Read the model definition and answer for the solid it produces. Units are mm, in the model's axes. A direction names the side the tool comes from. Round coordinates to 2 decimals unless told otherwise and drop trailing zeros. Order: outer loops, then holes, each group sorted by start corner. A loop starts at its lowest first (then second) coordinate and runs counter-clockwise, first axis right, second up. Notation, with made-up numbers: (-13.5, -34.75) - (8.5, -34.75) arc R36 ccw to (8.5, 2.25) - close; hole circle Ø5 at (63, 32). An arc over 180 degrees is marked (long way). One line per question, with ' | ' between items. Start each with the question number.
1) For faces 4 (the flat face through (368, 71, 95)), 5 (the cylindrical face through (377.75, 40.77, 85.56)), determine the directions among +Z, -Z, +X, -X, +Y, -Y from which every point of the face is accessible in a straight line to the end or side of a thin tool.
2) Straight lines are drawn through the part: line 1 (Z direction, x = 378.25, y = 114.8); line 2 (Y direction, x = 377.5, z = 13.2); line 3 (Z direction, x = 372.75, y = 40.7). For each, find the intervals that lie inside material, in ascending order. Write a range as from..to.
3) The part is cut by section A-A, the plane y = 114.8. Give the vertices of the cut face in (x, z), plus the area to 3 significant figures.
4) The mould has two halves that part along Y. Classify faces 1 (the flat face through (368, 22.5, 52)), 2 (the cylindrical face through (377.746, 116.426, 12.987)), 3 (the flat face through (388, 71, 53)): pulls with the +Y half, pulls with the -Y half, needs draft (parallel to the pull), parting line crosses it, or undercut.
5) The part is cut by section B-B, the plane z = 13.2. Give the vertices of the cut face in (x, y).
6) A flat-ended cylindrical pin translates along its axis: pin 1 (3 mm diameter, centred on y = 114.8, z = 13.2, fed in from +X). Find the tip coordinate at first contact, or state that the pin passes through.
from build123d import *

# Parameters (mm, degrees)
CYLINDER001_R     = 1.64
CYLINDER001_DEPTH = 50
CYLINDER_R        = 1.64
CYLINDER_DEPTH    = 50
BOX067_W          = 95.5
BOX067_H          = 85
BOX067_DEPTH      = 41.4


with BuildPart() as cylinder001:
    # Cylinder001 → Cylinder001 (new body)
    with BuildSketch(Plane(origin=(417.2, 114.8, 13.2), x_dir=(0, 0, 1), z_dir=(-1, 0, 0))):
        Circle(CYLINDER001_R)
    extrude(amount=CYLINDER001_DEPTH)


with BuildPart() as cylinder:
    # Cylinder → Cylinder (new body)
    with BuildSketch(Plane(origin=(417.2, 40.7, 87.2), x_dir=(0, 0, 1), z_dir=(-1, 0, 0))):
        Circle(CYLINDER_R)
    extrude(amount=CYLINDER_DEPTH)


with BuildPart() as cut002:
    # Box067 → Box067 (new body)
    with BuildSketch(Plane(origin=(388, 118, 10), x_dir=(0, -1, 0), z_dir=(-1, 0, 0))):
        with Locations((47.75, 42.5)):
            Rectangle(BOX067_W, BOX067_H)
    extrude(amount=BOX067_DEPTH)

    # Cut001: cut Cylinder
    add(cylinder.part, mode=Mode.SUBTRACT)

    # Cut002: cut Cylinder001
    add(cylinder001.part, mode=Mode.SUBTRACT)


solid = cut002.part
Values:
1) face 4: +Z, +X, -X, +Y, -Y | face 5: +X
2) line 1: z = 10..11.56, 14.84..95 | line 2: y = 22.5..113.16, 116.44..118 | line 3: z = 10..85.56, 88.84..95
3) outline: (346.6, 10) - (388, 10) - (388, 11.56) - (367.2, 11.56) - (367.2, 14.84) - (388, 14.84) - (388, 95) - (346.6, 95) - close | area: 3,450 mm^2
4) face 1: pulls with the -Y half | face 2: undercut | face 3: needs draft
5) outline: (346.6, 22.5) - (388, 22.5) - (388, 113.16) - (367.2, 113.16) - (367.2, 116.44) - (388, 116.44) - (388, 118) - (346.6, 118) - close
6) pin 1: stops at x = 367.2
